Build history of the part. All positions in model axes, mm. A direction names the side the tool comes from. Coordinates: 2 decimals unless noted, no trailing zeros. Write each loop counter-clockwise with the first axis right and the second up, starting at its lowest first coordinate (ties: lowest second). Pieces come first, ordered by that corner, then holes. Notation, with made-up numbers: (-35.75, 31) -> (-1.75, 31) arc R30 ccw to (-1.75, 70) -> close; hole circle Ø6 at (64, 63). An arc over 180 degrees is marked (long way). Write each question's results on one line, items separated by ' | '. Start each with the question number.
Q1. Tool access for faces 1 (the face through (-15.203, 8.446, 0.672)), 2 (the face through (-29, 0, 2.5)), 3 (the face through (23.1, 9.9, 14.3)): list every direction of +Z, -Z, +X, -X, +Y, -Y with a clear straight run to the whole face (end or side of a thin tool).
Q2. Saw through at B-B on x = 17.5. Give the cut face in (y, z), and give its area (3 significant figures).
Q3. Drill centre lines: line 1 (Y direction, x = -14, z = 0); line 2 (X direction, y = 6, z = -8); line 3 (Z direction, x = -14.4, y = -4.75). Where is each one in solid material? Low to high.
Q4. Two-plate mould, pull along Z, no slides. Class faces 4 (the face through (-12.61, -4.67, -8.43)), 5 (the face through (23.569, 13, 11)), 6 (the face through (-27, 0, -3)), 7 (the face through (-12.6, 9.3, 0)): released by +Z, released by -Z, zero draft, split by the parting line, or undercut.
Q5. Saw through at A-A on x = -16. Give the cut face in (y, z).
Q6. Drop flat-ended pins along their axis: pin 1 Ø3.5 at (y, z) = (11.5, 12) entering from -X; pin 2 Ø3 at (x, z) = (-11, 10) entering from -Y; pin 3 Ø4 at (x, z) = (-14.5, -8.5) entering from -Y; pin 4 Ø7.5 at (y, z) = (2, 6) entering from +X. Give the stop position or say it passes through.
from build123d import *

# Parameters (mm, degrees)
HOLE_WIZARD_M3_1_D       = 2.5
HOLE_WIZARD_M3_1_DEPTH   = 4
HOLE_WIZARD_M3_1_TIP     = 0.751075774
CUT_EXTRUDE_1_DEPTH      = 10
CUT_EXTRUDE_1_DEPTH_BACK = 10
SKETCH_4_R               = 1.5
SKETCH_5_W               = 6.291710533
SKETCH_5_H               = 14.520159288
CUT_EXTRUDE_2_DEPTH      = 11.5
HOLE_WIZARD_M3_2_D       = 2.5
HOLE_WIZARD_M3_2_DEPTH   = 5.5
HOLE_WIZARD_M3_2_TIP     = 0.751075774
EXTRUDE_2_DEPTH          = 10
EXTRUDE_2_DEPTH_BACK     = 10
SKETCH_9_W               = 3
SKETCH_9_H               = 10
FILLET_2_R               = 1.5


with BuildPart() as part:
    # 草图1 → 旋转1 (revolve)
    with BuildSketch(Plane.XY, mode=Mode.PRIVATE) as revolve_1_sk:
        Polygon((-34.231351781, 0), (-34.231351781, 3), (-19.831351781, 3), (-19.831351781, 6.5), (-17.231351781, 6.5), (-17.231351781, 12.2), (33.568648219, 12.2), (33.568648219, 3), (37.568648219, 3), (37.568648219, 0), align=None)
    revolve(revolve_1_sk.sketch.rotate(Axis((-36.151898734, 0, 0), (1, 0, 0)), 90), axis=Axis((-36.151898734, 0, 0), (1, 0, 0)))

    # M3 螺纹孔1
    with Locations(Plane(origin=(-17.231351781, 9.5, 0), x_dir=(0, 0, -1), z_dir=(-1, 0, 0))):
        with Locations((0, 0), (8.227241336, 14.25), (-8.227241336, 14.25)):
            Hole(HOLE_WIZARD_M3_1_D / 2, depth=HOLE_WIZARD_M3_1_DEPTH)
            with Locations((0, 0, -(HOLE_WIZARD_M3_1_DEPTH + HOLE_WIZARD_M3_1_TIP / 2))):  # 118° drill point
                Cone(0, HOLE_WIZARD_M3_1_D / 2, HOLE_WIZARD_M3_1_TIP, mode=Mode.SUBTRACT)

    # 草图4 → 切除-拉伸1 (cut, two sides: drawn at the far end of the back side and taken through both)
    with BuildSketch(Plane(origin=(0, 0, 0), x_dir=(1, 0, 0), z_dir=(0, 1, 0)).offset(-CUT_EXTRUDE_1_DEPTH_BACK)):
        with Locations(Location((-25.231351781, 0, 0), (0, 0, 90))):
            Circle(SKETCH_4_R)
    extrude(amount=CUT_EXTRUDE_1_DEPTH + CUT_EXTRUDE_1_DEPTH_BACK, mode=Mode.SUBTRACT)

    # 草图5 → 切除-拉伸2 (cut)
    with BuildSketch(Plane.ZY.offset(34.231351781)):
        with Locations((5.645855266, 0)):
            Rectangle(SKETCH_5_W, SKETCH_5_H)
    extrude(amount=-CUT_EXTRUDE_2_DEPTH, mode=Mode.SUBTRACT)

    # M3 螺纹孔2
    with Locations(Plane.ZY.offset(34.231351781)):
        with Locations((0, 0)):
            Hole(HOLE_WIZARD_M3_2_D / 2, depth=HOLE_WIZARD_M3_2_DEPTH)
            with Locations((0, 0, -(HOLE_WIZARD_M3_2_DEPTH + HOLE_WIZARD_M3_2_TIP / 2))):  # 118° drill point
                Cone(0, HOLE_WIZARD_M3_2_D / 2, HOLE_WIZARD_M3_2_TIP, mode=Mode.SUBTRACT)

    # 草图9 → 凸台-拉伸2 (add, two sides: drawn at the far end of the back side and taken through both)
    with BuildSketch(Plane(origin=(0, 9.345742206, 7.842008838), x_dir=(1, 0, 0), z_dir=(0, 0.7660444431189817, 0.642787609686535)).offset(-EXTRUDE_2_DEPTH_BACK)):
        with Locations((22.068648219, 0)):
            Rectangle(SKETCH_9_W, SKETCH_9_H)
    extrude(amount=EXTRUDE_2_DEPTH + EXTRUDE_2_DEPTH_BACK)

    # 圆角2
    fillet_2_edges = [part.edges().sort_by_distance(p)[0] for p in [
        (23.568648219, 9.55155762, 14.541744923),
        (20.568648219, 9.55155762, 14.541744923),
        (23.568648219, 15.979433717, 6.881300491),
        (20.568648219, 15.979433717, 6.881300491),
    ]]
    fillet(fillet_2_edges, radius=FILLET_2_R - 0.0001)  # a hair under: the kernel refuses the full size


solid = part.part
Returned:
1) face 1: -X | face 2: +Z, -X, +Y, -Y | face 3: +Z, +X
2) outline: circle Ø24.4 at (0, 0) | area: 468 mm2
3) line 1: y = -12.2 to 8.25, 10.75 to 12.2 | line 2: x = -17.23 to 33.57 | line 3: z = -11.24 to -9.48, -6.98 to 6.98, 9.48 to 11.24
4) face 4: undercut | face 5: zero draft | face 6: split by the parting line | face 7: undercut
5) outline: circle Ø24.4 at (0, 0); hole circle Ø2.5 at (-4.75, -8.23); hole circle Ø2.5 at (-4.75, 8.23); hole circle Ø2.5 at (9.5, 0)
6) pin 1: stops at x = 20.57 | pin 2: stops at y = -8.75 | pin 3: stops at y = -10.32 | pin 4: stops at x = 37.57
